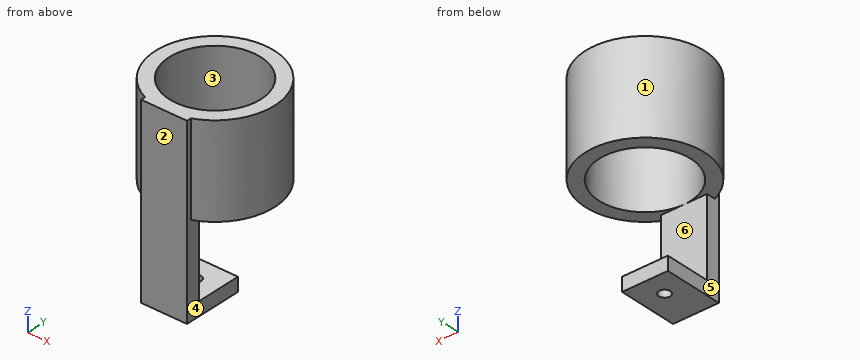
```python
from build123d import *

# Parameters (mm, degrees)
SKETCH1_W           = 12.7
SKETCH1_H           = 50.8
BOSS_EXTRUDE1_DEPTH = 3.81
SKETCH2_R           = 16.51
SKETCH2_R_2         = 12.7
BOSS_EXTRUDE2_DEPTH = 25.4
SKETCH3_W           = 12.7
SKETCH3_H           = 12.7
SKETCH3_R           = 1.5875
BOSS_EXTRUDE3_DEPTH = 3.81


with BuildPart() as part:
    # Sketch1 → Boss-Extrude1 (new body)
    with BuildSketch(Plane(origin=(0, 0, 0), x_dir=(1, 0, 0), z_dir=(0, 1, 0))):
        with Locations((6.35, 25.4)):
            Rectangle(SKETCH1_W, SKETCH1_H)
    extrude(amount=BOSS_EXTRUDE1_DEPTH)

    # Sketch2 → Boss-Extrude2 (add)
    with BuildSketch(Plane.XY):
        with Locations((6.35, 16.51)):
            Circle(SKETCH2_R)
        with Locations((6.35, 16.51)):
            Circle(SKETCH2_R_2, mode=Mode.SUBTRACT)
    extrude(amount=-BOSS_EXTRUDE2_DEPTH)

    # Sketch3 → Boss-Extrude3 (add)
    with BuildSketch(Plane(origin=(0, 0, -50.8), x_dir=(-1, 0, 0), z_dir=(0, 0, -1))):
        with Locations((-6.35, 10.16)):
            Rectangle(SKETCH3_W, SKETCH3_H)
        with Locations((-6.35, 10.16)):
            Circle(SKETCH3_R, mode=Mode.SUBTRACT)
    extrude(amount=-BOSS_EXTRUDE3_DEPTH)


solid = part.part
```
Design review of the part built by this model. Coordinates are the model's own, in mm. Face numbers are marked on the shaded views. A direction names the side the tool comes from. Coordinates: 2 decimals unless noted, no trailing zeros. Write each loop counter-clockwise with the first axis right and the second up, starting at its lowest first coordinate (ties: lowest second). Pieces come first, ordered by that corner, then holes. Notation, with made-up numbers: M 60,15.25 L 101,15.25 A20 ccw 101,42.25 Z; hole C 26.25,14 d8. An arc over 180 degrees is marked long. Answer as a JSON object with one key per item and string values.
Item 1: Machinability: for the marked faces 4, 5 and 6, which of the approach directions +Z, -Z, +X, -X, +Y, -Y give a long, thin tool a straight path to every point of the face, cutting with its end or side? Answer none if there is none.
Outcome:
{"face 4": "-Z, +X, -Y", "face 5": "-Z, -X, -Y", "face 6": "+X, -X, +Y"}
Item 2: Insertion check: pin 1 Ø3 at (x, z) = (6, -48.5) entering from +Y; pin 2 Ø4 at (x, y) = (6.35, 10.16) entering from +Z; pin 3 Ø6 at (x, y) = (18, 16) entering from -Z. Each pin has a flat end and moves straight along its axis. Give the tip position at first contact, or say it passes through.
Outcome:
{"pin 1": "y = 16.51", "pin 2": "z = -46.99", "pin 3": "z = -25.4"}
Item 3: Wall thickness on probe 1 along X at (y, z) = (10, -48); probe 2 along Y at (x, z) = (6.35, -49.4); probe 3 along X at (y, z) = (16, -20): over which ranges is each line inside the solid? List them lowest first.
Outcome:
{"probe 1": "0 to 4.77, 7.93 to 12.7", "probe 2": "0 to 8.57, 11.75 to 16.51", "probe 3": "-10.15 to -6.34, 19.04 to 22.85"}
Item 4: Add section C-C, the plane y = 8. Give the boundary of the cut face in (x, z), and give its area (3 significant figures).
Outcome:
{"outline": "M -7.8,-25.4 L -3.08,-25.4 L -3.08,0 L -7.8,0 Z; M 0,-50.8 L 12.7,-50.8 L 12.7,-46.99 L 0,-46.99 Z; M 15.78,-25.4 L 20.5,-25.4 L 20.5,0 L 15.78,0 Z", "area": "288 mm²"}
Item 5: Draft analysis for pull direction X (two halves, no side actions). For the marked faces 1, 2 and 3, state which applies: pulls with the +X half, pulls with the -X half, needs draft (parallel to the pull), parting line crosses it, or undercut.
Outcome:
{"face 1": "parting line crosses it", "face 2": "needs draft", "face 3": "undercut"}
Item 6: Add section B-B, the plane x = 14. Give the boundary of the cut face in (y, z), and give its area (3 significant figures).
Outcome:
{"outline": "M 1.88,-25.4 L 6.37,-25.4 L 6.37,0 L 1.88,0 Z; M 26.65,-25.4 L 31.14,-25.4 L 31.14,0 L 26.65,0 Z", "area": "228 mm²"}
Item 7: Add section A-A, the plane z = -4. Give the boundary of the cut face in (x, y).
Outcome:
{"outline": "M 0,0 L 12.7,0 L 12.7,1.27 A16.51 ccw long 0,1.27 Z; hole C 6.35,16.51 d25.4"}
Item 8: Add section D-D, the plane y = 19. Give the boundary of the cut face in (x, z).
Outcome:
{"outline": "M -9.97,-25.4 L -6.1,-25.4 L -6.1,0 L -9.97,0 Z; M 18.8,-25.4 L 22.67,-25.4 L 22.67,0 L 18.8,0 Z"}
